from build123d import *

# Parameters (mm, degrees)
SKETCH_1_W          = 85
SKETCH_1_H          = 80
EXTRUDE_1_DEPTH     = 10
SKETCH_2_R          = 5
SKETCH_2_R_2        = 2
CUT_EXTRUDE_1_DEPTH = 1
SKETCH_2_2_R        = 2
CUT_EXTRUDE_2_DEPTH = 78.419437026
SKETCH_3_R          = 15
CUT_EXTRUDE_3_DEPTH = 5
FILLET_1_R          = 0.5
FILLET_2_R          = 2
FILLET_3_R          = 2


with BuildPart() as part:
    # 草图1 → 凸台-拉伸1 (new body)
    with BuildSketch(Plane(origin=(0, 0, 0), x_dir=(1, 0, 0), z_dir=(0, 1, 0))):
        with Locations((-2.744934646, 22.021489166)):
            Rectangle(SKETCH_1_W, SKETCH_1_H)
    extrude(amount=EXTRUDE_1_DEPTH)

    # 草图2 → 切除-拉伸1 (cut)
    # profile 1 of 6: a face of its own
    with BuildSketch(Plane(origin=(0, 10, 0), x_dir=(1, 0, 0), z_dir=(0, 1, 0))):
        with Locations(Location((-2.744934646, 42.021489166, 0), (0, 0, 270))):
            Circle(SKETCH_2_R)
        with Locations(Location((-2.744934646, 42.021489166, 0), (0, 0, 270))):
            Circle(SKETCH_2_R_2, mode=Mode.SUBTRACT)
    # profile 2 of 6: a face of its own
    with BuildSketch(Plane(origin=(0, 10, 0), x_dir=(1, 0, 0), z_dir=(0, 1, 0))):
        with Locations(Location((-2.744934646, 2.021489166, 0), (0, 0, 270))):
            Circle(SKETCH_2_R)
        with Locations(Location((-2.744934646, 2.021489166, 0), (0, 0, 270))):
            Circle(SKETCH_2_R_2, mode=Mode.SUBTRACT)
    # profile 3 of 6: a face of its own
    with BuildSketch(Plane(origin=(0, 10, 0), x_dir=(1, 0, 0), z_dir=(0, 1, 0))):
        with Locations(Location((-23.994934646, 2.021489166, 0), (0, 0, 270))):
            Circle(SKETCH_2_R)
        with Locations(Location((-23.994934646, 2.021489166, 0), (0, 0, 270))):
            Circle(SKETCH_2_R_2, mode=Mode.SUBTRACT)
    # profile 4 of 6: a face of its own
    with BuildSketch(Plane(origin=(0, 10, 0), x_dir=(1, 0, 0), z_dir=(0, 1, 0))):
        with Locations(Location((18.505065354, 2.021489166, 0), (0, 0, 270))):
            Circle(SKETCH_2_R)
        with Locations(Location((18.505065354, 2.021489166, 0), (0, 0, 270))):
            Circle(SKETCH_2_R_2, mode=Mode.SUBTRACT)
    # profile 5 of 6: a face of its own
    with BuildSketch(Plane(origin=(0, 10, 0), x_dir=(1, 0, 0), z_dir=(0, 1, 0))):
        with Locations(Location((18.505065354, 42.021489166, 0), (0, 0, 270))):
            Circle(SKETCH_2_R)
        with Locations(Location((18.505065354, 42.021489166, 0), (0, 0, 270))):
            Circle(SKETCH_2_R_2, mode=Mode.SUBTRACT)
    # profile 6 of 6: a face of its own
    with BuildSketch(Plane(origin=(0, 10, 0), x_dir=(1, 0, 0), z_dir=(0, 1, 0))):
        with Locations(Location((-23.994934646, 42.021489166, 0), (0, 0, 270))):
            Circle(SKETCH_2_R)
        with Locations(Location((-23.994934646, 42.021489166, 0), (0, 0, 270))):
            Circle(SKETCH_2_R_2, mode=Mode.SUBTRACT)
    extrude(amount=-CUT_EXTRUDE_1_DEPTH, mode=Mode.SUBTRACT)

    # 草图2<2> → 切除-拉伸2 (cut, through all)
    with BuildSketch(Plane(origin=(0, 10, 0), x_dir=(1, 0, 0), z_dir=(0, 1, 0))):
        with Locations(Location((18.505065354, 42.021489166, 0), (0, 0, 270))):
            Circle(SKETCH_2_2_R)
        with Locations(Location((-2.744934646, 42.021489166, 0), (0, 0, 270))):
            Circle(SKETCH_2_2_R)
        with Locations(Location((-23.994934646, 42.021489166, 0), (0, 0, 270))):
            Circle(SKETCH_2_2_R)
        with Locations(Location((-23.994934646, 2.021489166, 0), (0, 0, 270))):
            Circle(SKETCH_2_2_R)
        with Locations(Location((-2.744934646, 2.021489166, 0), (0, 0, 270))):
            Circle(SKETCH_2_2_R)
        with Locations(Location((18.505065354, 2.021489166, 0), (0, 0, 270))):
            Circle(SKETCH_2_2_R)
    extrude(amount=-CUT_EXTRUDE_2_DEPTH, mode=Mode.SUBTRACT)

    # 草图3 → 切除-拉伸3 (cut)
    with BuildSketch(Plane(origin=(0, 0, 0), x_dir=(-1, 0, 0), z_dir=(0, -1, 0))):
        with Locations(Location((2.744934646, 22.021489166, 0), (0, 0, 90))):
            Circle(SKETCH_3_R)
    extrude(amount=-CUT_EXTRUDE_3_DEPTH, mode=Mode.SUBTRACT)

    # 圆角1
    fillet_1_edges = [part.edges().sort_by_distance(p)[0] for p in [
        (-2.744934646, 0, -7.021489166),
    ]]
    fillet(fillet_1_edges, radius=FILLET_1_R)

    # 圆角2
    fillet_2_edges = [part.edges().sort_by_distance(p)[0] for p in [
        (-2.744934646, 0, -62.021489166),
        (39.755065354, 0, -22.021489166),
        (-2.744934646, 0, 17.978510834),
        (-45.244934646, 0, -22.021489166),
    ]]
    fillet(fillet_2_edges, radius=FILLET_2_R)

    # 圆角3
    fillet_3_edges = [part.edges().sort_by_distance(p)[0] for p in [
        (39.755065354, 10, -22.021489166),
        (-2.744934646, 10, -62.021489166),
        (-45.244934646, 10, -22.021489166),
        (-2.744934646, 10, 17.978510834),
    ]]
    fillet(fillet_3_edges, radius=FILLET_3_R)


solid = part.part
Part model, mm, in its own coordinate system. A direction names the side the tool comes from. Coordinates: 2 decimals unless noted, no trailing zeros. Loops run counter-clockwise (first coordinate to the right, second up) from the corner with the lowest first, then second, coordinate; pieces in that order, holes last. Notation, with made-up numbers: (16, 16.5) -> (35, 16.5) arc R37 ccw to (35, 54.5) -> close; hole circle Ø8 at (80, -27.75). An arc over 180 degrees is marked (long way). Use a Markdown table: item, result. Add a question column.
Item 1: Which spindle directions (+Z, -Z, +X, -X, +Y, -Y) get a long thin tool onto all of the face, cutting with end or side? Do faces 4 (the cylindrical face through (18.59, 4.56, -4.02)), 5 (the cylindrical face through (-8.49, 2.718, -35.878)), 6 (the cylindrical face through (20.007, 9.507, -37.252)). Say none if no direction does.
Item 2: Probe probe 1 along Z at (x, y) = (-4.5, 1); probe 2 along Z at (x, y) = (18, 4.25); probe 3 along Z at (x, y) = (17.5, 3.5). List the from-to ranges inside material, lowest first.
Item 3: Pull direction X, two halves, no side cores. Call faces 1 (the cylindrical face through (39.185, 9.399, -22.581)), 2 (the flat face through (-3, 10, -23)), 3 (the flat face through (-3, 5, -22)): +X half, -X half, draft (parallel to the pull), parting line (faces both ways), or undercut.
Item 4: Flat gauge pins, fed straight in: P1, Ø2.5, axis at x = -2.74, z = -2.02, coming from the +Y side; P2, Ø15, axis at x = 3, z = -23.5, coming from the -Y side; P3, Ø5, axis at x = -3.5, z = -1, coming from the +Y side. Where does each tip first touch, or does it go through?
Item 5: Band-saw the part on A-A on y = 4. Write the cut outline in (x, z), plus the area to 3 significant figures.
Geometry says:
| question | item | result |
|---|---|---|
| 1 | face 4 | +Y, -Y |
| 1 | face 5 | -Y |
| 1 | face 6 | +Y |
| 2 | probe 1 | -61.75 to -42.98, -41.06 to -36.92, -7.12 to -2.98, -1.06 to 17.71 |
| 2 | probe 2 | -62.02 to -43.96, -40.09 to -3.96, -0.09 to 17.98 |
| 2 | probe 3 | -62.02 to -43.75, -40.29 to -3.75, -0.29 to 17.98 |
| 3 | face 1 | +X half |
| 3 | face 2 | draft |
| 3 | face 3 | undercut |
| 4 | P1 | through |
| 4 | P2 | y = 5 |
| 4 | P3 | y = 9 |
| 5 | outline | (-45.24, -62.02) -> (39.76, -62.02) -> (39.76, 17.98) -> (-45.24, 17.98) -> close; hole circle Ø4 at (-23.99, -42.02); hole circle Ø4 at (-23.99, -2.02); hole circle Ø30 at (-2.74, -22.02); hole circle Ø4 at (-2.74, -42.02); hole circle Ø4 at (-2.74, -2.02); hole circle Ø4 at (18.51, -42.02); hole circle Ø4 at (18.51, -2.02) |
| 5 | area | 6,020 mm² |
